from build123d import *

# Parameters (mm, degrees)
SKETCH_1_W      = 145
SKETCH_1_H      = 130
SKETCH_1_R      = 2.25
SKETCH_1_R_2    = 2.75
EXTRUDE_1_DEPTH = 1.5


with BuildPart() as part:
    # Эскиз1 → Вытянуть1 (new body)
    with BuildSketch(Plane.XY):
        Rectangle(SKETCH_1_W, SKETCH_1_H)
        with Locations((-67.5, 60)):
            Circle(SKETCH_1_R, mode=Mode.SUBTRACT)
        with Locations(Location((-67.5, -60, 0), (0, 0, 180))):
            Circle(SKETCH_1_R, mode=Mode.SUBTRACT)
        with Locations((67.5, -60)):
            Circle(SKETCH_1_R, mode=Mode.SUBTRACT)
        with Locations(Location((67.5, 60, 0), (0, 0, 180))):
            Circle(SKETCH_1_R, mode=Mode.SUBTRACT)
        with Locations((-52.5, 45)):
            Circle(SKETCH_1_R, mode=Mode.SUBTRACT)
        with Locations(Location((-52.5, -21, 0), (0, 0, 180))):
            Circle(SKETCH_1_R, mode=Mode.SUBTRACT)
        with Locations((-4.5, 45)):
            Circle(SKETCH_1_R, mode=Mode.SUBTRACT)
        with Locations(Location((-4.5, -21, 0), (0, 0, 180))):
            Circle(SKETCH_1_R, mode=Mode.SUBTRACT)
        with Locations((32.5, 15)):
            Circle(SKETCH_1_R_2, mode=Mode.SUBTRACT)
    extrude(amount=EXTRUDE_1_DEPTH)


solid = part.part
Verification items for the finished model (mm, model axes). Coordinates: 2 decimals unless noted, no trailing zeros. Write each loop counter-clockwise with the first axis right and the second up, starting at its lowest first coordinate (ties: lowest second). Pieces come first, ordered by that corner, then holes. Notation, with made-up numbers: M 60.5,31.25 L 118.5,31.25 A11 cw 118.5,43.25 Z; hole C 89,71 d2. An arc over 180 degrees is marked long. One line per question, with ' | ' between items.
1) Release check for a two-part mould opening along X. For faces 1 (the face through (-1, 1, 1.5)), 2 (the face through (65.714, -61.369, 0.74)) record: +X half, -X half, draft (parallel to the pull), parting line (faces both ways), or undercut.
Solutions:
face 1: draft | face 2: undercut
2) Sectioned sample at A-A on x = 67.5. Record the cut outline in (y, z), then the cut area to 4 significant figures.
Solutions:
outline: M -65,0 L -62.25,0 L -62.25,1.5 L -65,1.5 Z; M -57.75,0 L 57.75,0 L 57.75,1.5 L -57.75,1.5 Z; M 62.25,0 L 65,0 L 65,1.5 L 62.25,1.5 Z | area: 181.5 mm^2
3) Material ranges on L1, parallel to Y at x = -52.5, z = 0.4; L2, parallel to X at y = -21, z = 0.45; L3, parallel to Y at x = -67.5, z = 0.4, recorded low to high.
Solutions:
L1: -65 to -23.25, -18.75 to 42.75, 47.25 to 65 | L2: -72.5 to -54.75, -50.25 to -6.75, -2.25 to 72.5 | L3: -65 to -62.25, -57.75 to 57.75, 62.25 to 65
4) Sectioned sample at C-C on y = 60. Record the cut outline in (x, z).
Solutions:
outline: M -72.5,0 L -69.75,0 L -69.75,1.5 L -72.5,1.5 Z; M -65.25,0 L 65.25,0 L 65.25,1.5 L -65.25,1.5 Z; M 69.75,0 L 72.5,0 L 72.5,1.5 L 69.75,1.5 Z
5) Sectioned sample at D-D on x = 32.5. Record the cut outline in (y, z), then the cut area to 3 significant figures.
Solutions:
outline: M -65,0 L 12.25,0 L 12.25,1.5 L -65,1.5 Z; M 17.75,0 L 65,0 L 65,1.5 L 17.75,1.5 Z | area: 187 mm^2
6) Depth check by flat-ended pin: pin 1 Ø7 at (x, y) = (32.5, 15) entering from +Z; pin 2 Ø3.5 at (x, y) = (-52.5, 45) entering from +Z. Enter the tip coordinate at first touch or a pass-through.
Solutions:
pin 1: z = 1.5 | pin 2: through
7) Sectioned sample at B-B on y = 15. Record the cut outline in (x, z).
Solutions:
outline: M -72.5,0 L 29.75,0 L 29.75,1.5 L -72.5,1.5 Z; M 35.25,0 L 72.5,0 L 72.5,1.5 L 35.25,1.5 Z
